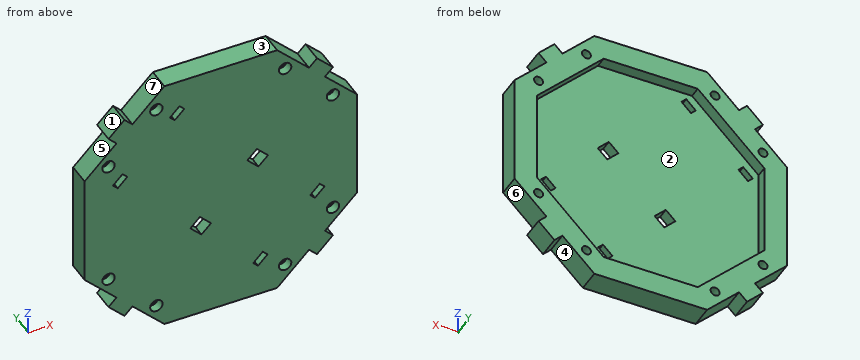
from build123d import *

# Parameters (mm, degrees)
BOSS_EXTRU_2_DEPTH                                   = 10
CHAMBRAGE_POUR_T_TE_CYLINDRIQUE_FENDUE_M_D           = 4
CHAMBRAGE_POUR_T_TE_CYLINDRIQUE_FENDUE_M_CBORE_D     = 5.5
CHAMBRAGE_POUR_T_TE_CYLINDRIQUE_FENDUE_M_CBORE_DEPTH = 4
ENL_V_MAT_EXTRU_1_DEPTH                              = 5
ENL_V_MAT_EXTRU_2_REACH                              = 87.502


with BuildPart() as part:
    # Esquisse1 → Boss.-Extru.2 (new body)
    with BuildSketch(Plane(origin=(0, 0, 0), x_dir=(1, 0, 0), z_dir=(0, 1, 0))):
        Polygon((60.355339059, 25), (25, 60.355339059), (-25, 60.355339059), (-60.355339059, 25), (-60.355339059, -25), (-25, -60.355339059), (25, -60.355339059), (60.355339059, -25), align=None)
        Polygon((39.142135624, 46.213203436), (46.213203436, 39.142135624), (49.748737342, 42.67766953), (42.67766953, 49.748737342), align=None)
        Polygon((49.748737342, -42.67766953), (46.213203436, -39.142135624), (39.142135624, -46.213203436), (42.67766953, -49.748737342), align=None)
        Polygon((-42.67766953, -49.748737342), (-39.142135624, -46.213203436), (-46.213203436, -39.142135624), (-49.748737342, -42.67766953), align=None)
        Polygon((-46.213203436, 39.142135624), (-39.142135624, 46.213203436), (-42.67766953, 49.748737342), (-49.748737342, 42.67766953), align=None)
    extrude(amount=BOSS_EXTRU_2_DEPTH)

    # Chambrage pour tête cylindrique fendue M31 (through all)
    with Locations(Plane(origin=(-49.748737342, 0, -28.535533906), x_dir=(0, 0, -1), z_dir=(0, -1, 0))):
        with Locations((0, 0), (21.213203436, 21.213203436), (21.213203436, 78.284271248), (0, 99.497474684), (-78.284271248, 78.284271248), (-57.071067812, 99.497474684), (-78.284271248, 21.213203436), (-57.071067812, 0)):
            CounterBoreHole(CHAMBRAGE_POUR_T_TE_CYLINDRIQUE_FENDUE_M_D / 2, CHAMBRAGE_POUR_T_TE_CYLINDRIQUE_FENDUE_M_CBORE_D / 2, CHAMBRAGE_POUR_T_TE_CYLINDRIQUE_FENDUE_M_CBORE_DEPTH)

    # Esquisse6 → Enlèv. mat.-Extru.1 (cut)
    with BuildSketch(Plane(origin=(0, 10, 0), x_dir=(1, 0, 0), z_dir=(0, 1, 0))):
        Polygon((20.857864376, 50.355339059), (-20.857864376, 50.355339059), (-50.355339059, 20.857864376), (-50.355339059, -20.857864376), (-20.857864376, -50.355339059), (20.857864376, -50.355339059), (50.355339059, -20.857864376), (50.355339059, 20.857864376), align=None)
    extrude(amount=-ENL_V_MAT_EXTRU_1_DEPTH, mode=Mode.SUBTRACT)

    # Esquisse7 → Enlèv. mat.-Extru.2 (cut, up to next)
    with BuildSketch(Plane(origin=(0, 5, 0), x_dir=(1, 0, 0), z_dir=(0, 1, 0)), mode=Mode.PRIVATE) as enl_v_mat_extru_2_sk1:
        Polygon((-47.779960262, -18.282485579), (-45.658639918, -16.161165235), (-41.415999231, -20.403805922), (-43.537319575, -22.525126266), align=None)
    enl_v_mat_extru_2_tool1 = extrude(enl_v_mat_extru_2_sk1.sketch, amount=-ENL_V_MAT_EXTRU_2_REACH, mode=Mode.PRIVATE) & part.part
    # Esquisse7 → Enlèv. mat.-Extru.2 (cut, up to next)
    with BuildSketch(Plane(origin=(0, 5, 0), x_dir=(1, 0, 0), z_dir=(0, 1, 0)), mode=Mode.PRIVATE) as enl_v_mat_extru_2_sk2:
        Polygon((-13.485281374, 16.012193309), (-8.535533906, 20.961940777), (-4.292893219, 16.71930009), (-9.242640687, 11.769552622), align=None)
    enl_v_mat_extru_2_tool2 = extrude(enl_v_mat_extru_2_sk2.sketch, amount=-ENL_V_MAT_EXTRU_2_REACH, mode=Mode.PRIVATE) & part.part
    # Esquisse7 → Enlèv. mat.-Extru.2 (cut, up to next)
    with BuildSketch(Plane(origin=(0, 5, 0), x_dir=(1, 0, 0), z_dir=(0, 1, 0)), mode=Mode.PRIVATE) as enl_v_mat_extru_2_sk3:
        Polygon((14.393398282, 43.890872965), (16.514718626, 46.012193309), (20.757359313, 41.769552622), (18.636038969, 39.648232278), align=None)
    enl_v_mat_extru_2_tool3 = extrude(enl_v_mat_extru_2_sk3.sketch, amount=-ENL_V_MAT_EXTRU_2_REACH, mode=Mode.PRIVATE) & part.part
    # Esquisse7 → Enlèv. mat.-Extru.2 (cut, up to next)
    with BuildSketch(Plane(origin=(0, 5, 0), x_dir=(1, 0, 0), z_dir=(0, 1, 0)), mode=Mode.PRIVATE) as enl_v_mat_extru_2_sk4:
        Polygon((-20.403805922, -41.415999231), (-22.525126266, -43.537319575), (-18.282485579, -47.779960262), (-16.161165235, -45.658639918), align=None)
    enl_v_mat_extru_2_tool4 = extrude(enl_v_mat_extru_2_sk4.sketch, amount=-ENL_V_MAT_EXTRU_2_REACH, mode=Mode.PRIVATE) & part.part
    # Esquisse7 → Enlèv. mat.-Extru.2 (cut, up to next)
    with BuildSketch(Plane(origin=(0, 5, 0), x_dir=(1, 0, 0), z_dir=(0, 1, 0)), mode=Mode.PRIVATE) as enl_v_mat_extru_2_sk5:
        Polygon((39.648232278, 18.636038969), (43.890872965, 14.393398282), (46.012193309, 16.514718626), (41.769552622, 20.757359313), align=None)
    enl_v_mat_extru_2_tool5 = extrude(enl_v_mat_extru_2_sk5.sketch, amount=-ENL_V_MAT_EXTRU_2_REACH, mode=Mode.PRIVATE) & part.part
    # Esquisse7 → Enlèv. mat.-Extru.2 (cut, up to next)
    with BuildSketch(Plane(origin=(0, 5, 0), x_dir=(1, 0, 0), z_dir=(0, 1, 0)), mode=Mode.PRIVATE) as enl_v_mat_extru_2_sk6:
        Polygon((16.71930009, -4.292893219), (11.769552622, -9.242640687), (16.012193309, -13.485281374), (20.961940777, -8.535533906), align=None)
    enl_v_mat_extru_2_tool6 = extrude(enl_v_mat_extru_2_sk6.sketch, amount=-ENL_V_MAT_EXTRU_2_REACH, mode=Mode.PRIVATE) & part.part
    add(enl_v_mat_extru_2_tool1.solids().sort_by_distance((-44.59798, 5, 19.343146))[0], mode=Mode.SUBTRACT)
    add(enl_v_mat_extru_2_tool2.solids().sort_by_distance((-8.889087, 5, -16.365747))[0], mode=Mode.SUBTRACT)
    add(enl_v_mat_extru_2_tool3.solids().sort_by_distance((17.575379, 5, -42.830213))[0], mode=Mode.SUBTRACT)
    add(enl_v_mat_extru_2_tool4.solids().sort_by_distance((-19.343146, 5, 44.59798))[0], mode=Mode.SUBTRACT)
    add(enl_v_mat_extru_2_tool5.solids().sort_by_distance((42.830213, 5, -17.575379))[0], mode=Mode.SUBTRACT)
    add(enl_v_mat_extru_2_tool6.solids().sort_by_distance((16.365747, 5, 8.889087))[0], mode=Mode.SUBTRACT)


solid = part.part
Geometry check sheet. Reference: the model listing, model coordinates, mm. Face numbers are marked on the shaded views. A direction names the side the tool comes from. Round coordinates to 2 decimals unless told otherwise and drop trailing zeros. Order: outer loops, then holes, each group sorted by start corner. A loop starts at its lowest first (then second) coordinate and runs counter-clockwise, first axis right, second up. Notation, with made-up numbers: M 71.5,17 L 123.5,17 A29 ccw 123.5,42 Z; hole C 27,11.25 d1. An arc over 180 degrees is marked long. Write each question's results on one line, items separated by ' | '. Start each with the question number.
1. Draft check along X on the marked faces 1, 2 and 3. Enter one of: pulls with the +X half, pulls with the -X half, needs draft (parallel to the pull), parting line crosses it, or undercut.
2. Material ranges on L1, parallel to Z at x = -19.5, y = 6.5; L2, parallel to X at y = 2.5, z = -20; L3, parallel to Z at x = -49.5, y = 9, recorded low to high. Write a range as from..to.
3. Cross-section at A-A on x = 6. Record the boundary of the cut face in (y, z).
4. Cross-section at C-C on y = 8.25. Give the number of separate pieces and of enclosed holes in the cut face, plus the area to 3 significant figures.
5. Set-up check for the marked faces 4, 5, 6 and 7: record each of +Z, -Z, +X, -X, +Y, -Y from which the full face is reachable in a straight line by a thin tool's end or side.
6. Go/stop test with flat-tipped pins: P1, Ø4.5, axis at x = 28.54, z = -49.75, coming from the -Y side; P2, Ø6, axis at x = -16.5, z = 29.5, coming from the +Y side. Record where each tip stops, or that it passes through.
7. Cross-section at B-B on z = -23.5. Record the boundary of the cut face in (x, y).
Resolved:
1) face 1: pulls with the -X half | face 2: undercut | face 3: needs draft
2) L1: -60.36..-50.36, 50.36..60.36 | L2: -60.36..-9.5, -7.57..41.01, 42.53..60.36 | L3: -42.93..-42.43, -35.86..-30.52, -26.55..-21.71, 21.71..26.55, 30.52..35.86, 42.43..42.93
3) outline: M 0,-60.36 L 10,-60.36 L 10,-50.36 L 5,-50.36 L 5,50.36 L 10,50.36 L 10,60.36 L 0,60.36 Z
4) separate pieces: 1 | enclosed holes: 9 | area: 3,770 mm2
5) face 4: -Z, +Y, -Y | face 5: -X, +Y, -Y | face 6: +X, +Y, -Y | face 7: +Z, +Y, -Y
6) P1: y = 4 | P2: y = 5
7) outline: M -60.36,0 L 60.36,0 L 60.36,10 L 47.71,10 L 47.71,5 L -47.71,5 L -47.71,10 L -60.36,10 Z
